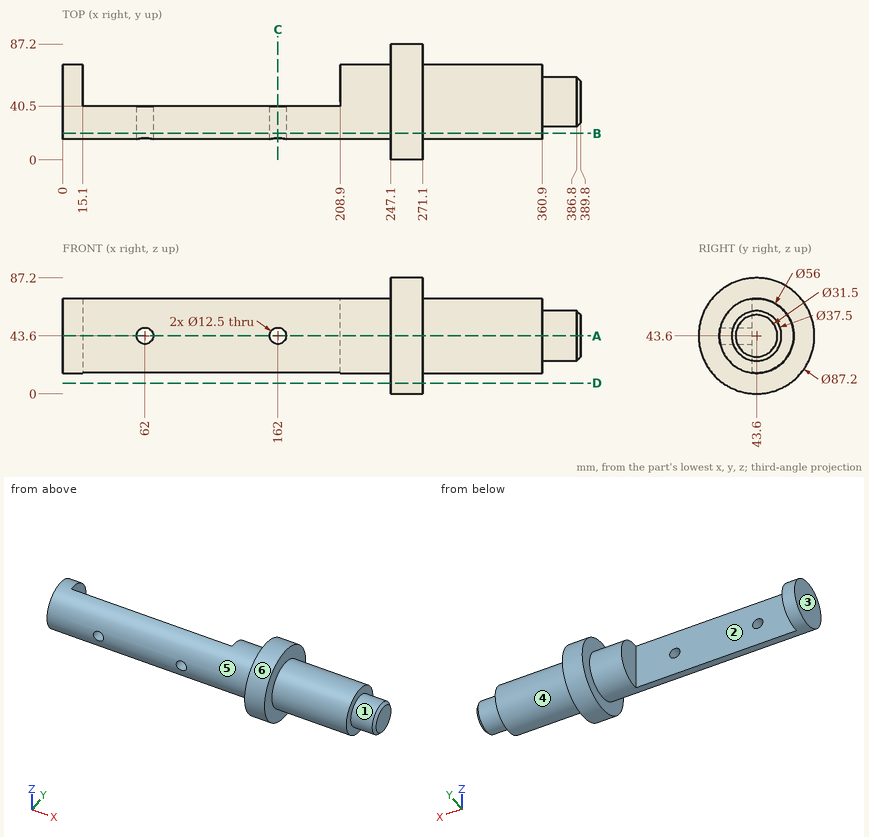
Verification items for this drawing (mm, ordinates from the low corner). A direction names the side the tool comes from. Round coordinates to 2 decimals unless told otherwise and drop trailing zeros. Loops run counter-clockwise (first coordinate to the right, second up) from the corner with the lowest first, then second, coordinate; pieces in that order, holes last. Notation, with made-up numbers: (3, 84.5) -> (11, 84.5) arc R20 cw to (11, 100.5) -> close; hole circle Ø7 at (84, 88). An arc over 180 degrees is marked (long way). Answer in a Markdown table with one row per item.
Q1. Thickness scan on L1, parallel to X at y = 32.25, z = 43.6; L2, parallel to X at y = 22.25, z = 43.6; L3, parallel to X at y = 46, z = 36.5. Record the ranges inside material, lowest first.
Data:
| item | result |
|---|---|
| L1 | x = 0 to 55.75, 68.25 to 155.75, 168.25 to 389.8 |
| L2 | x = 0 to 55.75, 68.25 to 155.75, 168.25 to 360.9 |
| L3 | x = 0 to 15.1, 208.9 to 389.8 |
Q2. Sectioned sample at B-B on y = 20. Enter the section's corners in (x, z).
Data:
| item | result |
|---|---|
| outline | (0, 28.53) -> (247.1, 28.53) -> (247.1, 6.94) -> (271.1, 6.94) -> (271.1, 28.53) -> (360.9, 28.53) -> (360.9, 58.67) -> (271.1, 58.67) -> (271.1, 80.26) -> (247.1, 80.26) -> (247.1, 58.67) -> (0, 58.67) -> close; hole circle Ø12.5 at (62, 43.6); hole circle Ø12.5 at (162, 43.6) |
Q3. Set-up check for the marked faces 4, 5 and 6: record each of +Z, -Z, +X, -X, +Y, -Y from which the full face is reachable in a straight line by a thin tool's end or side.
Data:
| item | result |
|---|---|
| face 4 | +X |
| face 5 | -X |
| face 6 | +X, -X |
Q4. Go/stop test with flat-tipped pins: P1, Ø5, axis at x = 131.5, z = 26.5, coming from the -Y side; P2, Ø1, axis at x = 230, z = 57, coming from the -Y side; P3, Ø6, axis at x = 282, z = 65, coming from the +Y side; P4, Ø10, axis at x = 162, z = 43.6, coming from the +Y side. Record where each tip stops, or that it passes through.
Data:
| item | result |
|---|---|
| P1 | stops at y = 19.71 |
| P2 | stops at y = 18.75 |
| P3 | stops at y = 64.71 |
| P4 | passes through |
Q5. Sectioned sample at D-D on z = 8. Enter the section's corners in (x, y).
Data:
| item | result |
|---|---|
| outline | (247.1, 18.43) -> (271.1, 18.43) -> (271.1, 68.77) -> (247.1, 68.77) -> close |
Q6. Release check for a two-part mould opening along X. For the marked faces 1, 2 and 3 record: released by +X, released by -X, zero draft, split by the parting line, or undercut.
Data:
| item | result |
|---|---|
| face 1 | zero draft |
| face 2 | undercut |
| face 3 | released by -X |
Q7. Sectioned sample at C-C on x = 162. Enter the section's corners in (y, z).
Data:
| item | result |
|---|---|
| outline | (16.31, 37.35) arc R28 ccw to (40.5, 15.77) -> (40.5, 37.35) -> close; (16.31, 49.85) -> (40.5, 49.85) -> (40.5, 71.43) arc R28 ccw to start |
Q8. Sectioned sample at A-A on z = 43.6. Give the number of separate pieces and of enclosed holes in the cut face, then the cut area to 3 significant figures.
Data:
| item | result |
|---|---|
| separate pieces | 3 |
| enclosed holes | 0 |
| area | 15,400 mm^2 |
